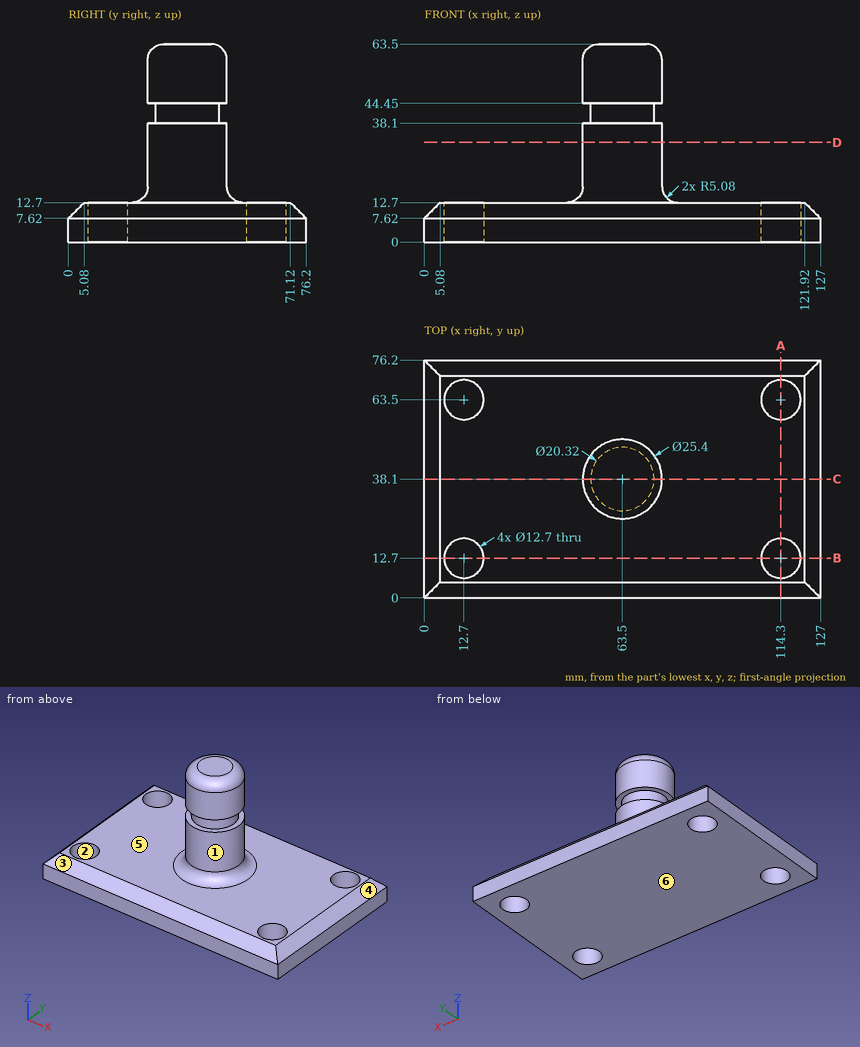
The figure shows three views and two pictorial views of one solid part (mm, origin at its lowest corner). Answer the questions. A direction names the side the tool comes from. Give positions to 0.01 mm unless a question says otherwise; leave off trailing zeros. Write each loop counter-clockwise with the first axis right and the second up, starting at its lowest first coordinate (ties: lowest second). Pieces come first, ordered by that corner, then holes. Notation, with made-up numbers: M 30.5,67 L 43.5,67 A22 cw 43.5,74 Z; hole C 77.25,87 d11. An arc over 180 degrees is marked long. One line per item, written item: value. Start each with the question number.
(1) A tool of negligible diameter and unlimited length cuts with its end or side. For the marked faces 5 and 6, from which of +Z, -Z, +X, -X, +Y, -Y can it reach the whole face along a straight path? Write none if from no direction.
(2) Find section D-D (z = 32). Determine the outline of the cut face in (x, y).
(3) Flat-ended cylindrical pins translate along their axes: pin 1 Ø5 at (y, z) = (38, 40) entering from +X; pin 2 Ø1.5 at (x, z) = (61, 54) entering from -Y; pin 3 Ø14.5 at (x, y) = (12.7, 12.7) entering from +Z; pin 4 Ø12 at (y, z) = (15.5, 32) entering from +X. Find the tip coordinate at first contact, or state that the pin passes through.
(4) Find section B-B (y = 12.7). Determine the outline of the cut face in (x, z).
(5) Find section C-C (y = 38.1). Determine the outline of the cut face in (x, z), plus the area to 3 significant figures.
(6) Determine the mould class of the marked faces 1, 2, 3 and 4 for opening direction X: pulls with the +X half, pulls with the -X half, needs draft (parallel to the pull), parting line crosses it, or undercut.
(7) Find the intervals of material crossed by line 1 (Y direction, x = 114.3, z = 4.5); line 2 (X direction, y = 63, z = 7); line 3 (X direction, y = 12, z = 9), in increasing order.
(8) Find section A-A (x = 114.3). Determine the outline of the cut face in (y, z).
Results below:
1. face 5: +Z
1. face 6: -Z, +X, -X, +Y, -Y
2. outline: C 63.5,38.1 d25.4
3. pin 1: stops at x = 76.2
3. pin 2: stops at y = 25.52
3. pin 3: stops at z = 12.7
3. pin 4: passes through
4. outline: M 0,0 L 6.35,0 L 6.35,12.7 L 5.08,12.7 L 0,7.62 Z; M 19.05,0 L 107.95,0 L 107.95,12.7 L 19.05,12.7 Z; M 120.65,0 L 127,0 L 127,7.62 L 121.92,12.7 L 120.65,12.7 Z
5. outline: M 0,0 L 127,0 L 127,7.62 L 121.92,12.7 L 81.28,12.7 A5.08 cw 76.2,17.78 L 76.2,38.1 L 73.66,38.1 L 73.66,44.45 L 76.2,44.45 L 76.2,58.42 A5.08 ccw 71.12,63.5 L 55.88,63.5 A5.08 ccw 50.8,58.42 L 50.8,44.45 L 53.34,44.45 L 53.34,38.1 L 50.8,38.1 L 50.8,17.78 A5.08 cw 45.72,12.7 L 5.08,12.7 L 0,7.62 Z
5. area: 2,850 mm^2
6. face 1: parting line crosses it
6. face 2: undercut
6. face 3: needs draft
6. face 4: pulls with the +X half
7. line 1: y = 0 to 6.35, 19.05 to 57.15, 69.85 to 76.2
7. line 2: x = 0 to 6.37, 19.03 to 107.97, 120.63 to 127
7. line 3: x = 1.38 to 6.39, 19.01 to 107.99, 120.61 to 125.62
8. outline: M 0,0 L 6.35,0 L 6.35,12.7 L 5.08,12.7 L 0,7.62 Z; M 19.05,0 L 57.15,0 L 57.15,12.7 L 19.05,12.7 Z; M 69.85,0 L 76.2,0 L 76.2,7.62 L 71.12,12.7 L 69.85,12.7 Z
